Design review of the part built by this model. Coordinates are the model's own, in mm. A direction names the side the tool comes from. Round coordinates to 2 decimals unless told otherwise and drop trailing zeros. Order: outer loops, then holes, each group sorted by start corner. A loop starts at its lowest first (then second) coordinate and runs counter-clockwise, first axis right, second up.
from build123d import *

# Parameters (mm, degrees)
SKETCH1_W                 = 75
SKETCH1_H                 = 35
BOSS_EXTRUDE1_DEPTH       = 67
CUT_EXTRUDE1_DEPTH        = 60
SKETCH4_W                 = 15
SKETCH4_H                 = 10
CUT_EXTRUDE2_DEPTH        = 73.886898686
SKETCH5_W                 = 22
SKETCH5_H                 = 3
CUT_EXTRUDE3_DEPTH        = 43
F_3_0MM_DOWEL_HOLE1_D     = 3.3
F_3_0MM_DOWEL_HOLE1_DEPTH = 10
F_3_0MM_DOWEL_HOLE1_TIP   = 0.991420021
SKETCH8_R                 = 2.65
CUT_EXTRUDE4_DEPTH        = 103.079625783
FILLET1_R                 = 4


with BuildPart() as part:
    # Sketch1 → Boss-Extrude1 (new body)
    with BuildSketch(Plane.XY):
        Rectangle(SKETCH1_W, SKETCH1_H)
    extrude(amount=-BOSS_EXTRUDE1_DEPTH)

    # Sketch2 → Cut-Extrude1 (cut)
    with BuildSketch(Plane(origin=(0, 0, -67), x_dir=(-1, 0, 0), z_dir=(0, 0, -1))):
        Polygon((-22.75, -17.5), (22.75, -17.5), (22.75, 8.5), (11, 14.5), (-11, 14.5), (-22.75, 8.5), align=None)
    extrude(amount=-CUT_EXTRUDE1_DEPTH, mode=Mode.SUBTRACT)

    # Sketch4 → Cut-Extrude2 (cut, through all)
    with BuildSketch(Plane(origin=(0, 0, -7), x_dir=(-1, 0, 0), z_dir=(0, 0, -1))):
        with Locations((0, -12.5)):
            Rectangle(SKETCH4_W, SKETCH4_H)
    extrude(amount=-CUT_EXTRUDE2_DEPTH, mode=Mode.SUBTRACT)

    # Sketch5 → Cut-Extrude3 (cut)
    with BuildSketch(Plane(origin=(0, 0, -67), x_dir=(-1, 0, 0), z_dir=(0, 0, -1))):
        with Locations((0, 16)):
            Rectangle(SKETCH5_W, SKETCH5_H)
    extrude(amount=-CUT_EXTRUDE3_DEPTH, mode=Mode.SUBTRACT)

    # Ø3.0mm Dowel Hole1
    with Locations(Plane(origin=(0, 17.5, 0), x_dir=(1, 0, 0), z_dir=(0, 1, 0))):
        with Locations((-31.04375, 31), (-31.04375, 42), (-20.13125, 42), (-20.13125, 31), (-5.5, 16.36875), (5.5, 16.36875), (-5.5, 5.45625), (5.5, 5.45625), (31.04375, 42), (20.13125, 42), (31.04375, 31), (20.13125, 31)):
            Hole(F_3_0MM_DOWEL_HOLE1_D / 2, depth=F_3_0MM_DOWEL_HOLE1_DEPTH)
            with Locations((0, 0, -(F_3_0MM_DOWEL_HOLE1_DEPTH + F_3_0MM_DOWEL_HOLE1_TIP / 2))):  # 118° drill point
                Cone(0, F_3_0MM_DOWEL_HOLE1_D / 2, F_3_0MM_DOWEL_HOLE1_TIP, mode=Mode.SUBTRACT)

    # Sketch8 → Cut-Extrude4 (cut, through all)
    with BuildSketch(Plane.ZY.offset(37.5)):
        with Locations((-61, -7.5)):
            Circle(SKETCH8_R)
        with Locations((-50, -7.5)):
            Circle(SKETCH8_R)
    extrude(amount=-CUT_EXTRUDE4_DEPTH, mode=Mode.SUBTRACT)

    # Fillet1
    # the kernel refuses this fillet: 4 mm, written as the material it takes off along each edge
    with BuildSketch(Plane(origin=(33.5, 13.5, -4), x_dir=(0, 0, 1), z_dir=(1, 0, 0))) as fillet1_piece_1_section:
        Polygon((0, 0), (FILLET1_R, 0), (FILLET1_R, -FILLET1_R), (0, -FILLET1_R), align=None)
    fillet1_piece_1 = extrude(amount=FILLET1_R, mode=Mode.PRIVATE)
    fillet1_piece_1 = fillet1_piece_1 - Plane(origin=(33.5, 13.5, -4), x_dir=(0, -0.7071067811865475, -0.7071067811865475), z_dir=(1, 0, 0)) * Sphere(FILLET1_R, mode=Mode.PRIVATE)
    add(fillet1_piece_1, mode=Mode.SUBTRACT)
    with BuildSketch(Plane(origin=(-33.5, 13.5, -4), x_dir=(-1, 0, 0), z_dir=(0, 0, 1))) as fillet1_piece_2_section:
        Polygon((0, 0), (FILLET1_R, 0), (FILLET1_R, -FILLET1_R), (0, -FILLET1_R), align=None)
    fillet1_piece_2 = extrude(amount=FILLET1_R, mode=Mode.PRIVATE)
    fillet1_piece_2 = fillet1_piece_2 - Plane(origin=(-33.5, 13.5, -4), x_dir=(0.7071067811865475, -0.7071067811865475, 0), z_dir=(0, 0, 1)) * Sphere(FILLET1_R, mode=Mode.PRIVATE)
    add(fillet1_piece_2, mode=Mode.SUBTRACT)
    with BuildSketch(Plane(origin=(-33.5, 13.5, -63), x_dir=(-1, 0, 0), z_dir=(0, 0, -1))) as fillet1_piece_3_section:
        Polygon((0, 0), (FILLET1_R, 0), (FILLET1_R, FILLET1_R), (0, FILLET1_R), align=None)
    fillet1_piece_3 = extrude(amount=FILLET1_R, mode=Mode.PRIVATE)
    fillet1_piece_3 = fillet1_piece_3 - Plane(origin=(-33.5, 13.5, -63), x_dir=(0.7071067811865475, -0.7071067811865475, 0), z_dir=(0, 0, -1)) * Sphere(FILLET1_R, mode=Mode.PRIVATE)
    add(fillet1_piece_3, mode=Mode.SUBTRACT)
    with BuildSketch(Plane(origin=(33.5, 13.5, -63), x_dir=(0, 1, 0), z_dir=(1, 0, 0))) as fillet1_piece_4_section:
        Polygon((0, 0), (FILLET1_R, 0), (FILLET1_R, -FILLET1_R), (0, -FILLET1_R), align=None)
    fillet1_piece_4 = extrude(amount=FILLET1_R, mode=Mode.PRIVATE)
    fillet1_piece_4 = fillet1_piece_4 - Plane(origin=(33.5, 13.5, -63), x_dir=(0, -0.7071067811865475, 0.7071067811865475), z_dir=(1, 0, 0)) * Sphere(FILLET1_R, mode=Mode.PRIVATE)
    add(fillet1_piece_4, mode=Mode.SUBTRACT)
    with BuildSketch(Plane(origin=(37.5, -27.5, 0), x_dir=(-1, 0, 0), z_dir=(0, 1, 0)), Plane(origin=(-37.5, 13.5, 0), x_dir=(1, 0, 0), z_dir=(0, -1, 0)), Plane(origin=(37.5, -27.5, -67), x_dir=(0, 0, 1), z_dir=(0, 1, 0))) as fillet1_piece_5:
        with BuildLine():
            CenterArc((FILLET1_R, -FILLET1_R), FILLET1_R, 90, 90)
            Line((0, -FILLET1_R), (0, 0))
            Line((0, 0), (FILLET1_R, 0))
        make_face()
    extrude(amount=41, mode=Mode.SUBTRACT)
    with BuildSketch(Plane(origin=(-37.5, 13.5, -67), x_dir=(1, 0, 0), z_dir=(0, -1, 0))) as fillet1_piece_6:
        with BuildLine():
            CenterArc((FILLET1_R, FILLET1_R), FILLET1_R, 180, 90)
            Line((0, FILLET1_R), (0, 0))
            Line((0, 0), (FILLET1_R, 0))
        make_face()
    extrude(amount=41, mode=Mode.SUBTRACT)
    with BuildSketch(Plane(origin=(-1, 17.5, -67), x_dir=(0, -1, 0), z_dir=(-1, 0, 0))) as fillet1_piece_7:
        with BuildLine():
            CenterArc((FILLET1_R, FILLET1_R), FILLET1_R, 180, 90)
            Line((0, FILLET1_R), (0, 0))
            Line((0, 0), (FILLET1_R, 0))
        make_face()
    extrude(amount=32.5, mode=Mode.SUBTRACT)
    with BuildSketch(Plane(origin=(33.5, 17.5, -67), x_dir=(0, 0, 1), z_dir=(-1, 0, 0))) as fillet1_piece_8:
        with BuildLine():
            CenterArc((FILLET1_R, -FILLET1_R), FILLET1_R, 90, 90)
            Line((0, -FILLET1_R), (0, 0))
            Line((0, 0), (FILLET1_R, 0))
        make_face()
    extrude(amount=32.5, mode=Mode.SUBTRACT)
    with BuildSketch(Plane(origin=(37.5, 17.5, -4), x_dir=(-1, 0, 0), z_dir=(0, 0, -1)), Plane(origin=(-37.5, 17.5, -4), x_dir=(0, -1, 0), z_dir=(0, 0, -1))) as fillet1_piece_9:
        with BuildLine():
            CenterArc((FILLET1_R, -FILLET1_R), FILLET1_R, 90, 90)
            Line((0, -FILLET1_R), (0, 0))
            Line((0, 0), (FILLET1_R, 0))
        make_face()
    extrude(amount=59, mode=Mode.SUBTRACT)
    with BuildSketch(Plane(origin=(33.5, 17.5, 0), x_dir=(0, -1, 0), z_dir=(-1, 0, 0))) as fillet1_piece_10:
        with BuildLine():
            CenterArc((FILLET1_R, -FILLET1_R), FILLET1_R, 90, 90)
            Line((0, -FILLET1_R), (0, 0))
            Line((0, 0), (FILLET1_R, 0))
        make_face()
    extrude(amount=67, mode=Mode.SUBTRACT)


solid = part.part
1) Take a section at D-D on y = 3.5. Give the boundary of the cut face in (x, z).
Results:
outline: (-37.5, -63) arc R4 ccw to (-33.5, -67) - (-22.75, -67) - (-22.75, -7) - (22.75, -7) - (22.75, -67) - (33.5, -67) arc R4 ccw to (37.5, -63) - (37.5, -4) arc R4 ccw to (33.5, 0) - (-33.5, 0) arc R4 ccw to (-37.5, -4) - close
2) To check wall thickness, follow line 1 along X through (y, z) = (-7, -39.5); line 2 along X through (y, z) = (8, -43.5); line 3 along Z through (x, y) = (-31, -6). State the ranges of each line that lie inside material, in increasing order.
Results:
line 1: x = -37.5 to -22.75, 22.75 to 37.5
line 2: x = -37.5 to -31.73, -30.36 to -22.75, 22.75 to 30.36, 31.73 to 37.5
line 3: z = -67 to -63.18, -58.82 to -52.18, -47.82 to 0
3) For faces 1 (the face through (16.793, 11.542, -37.42)), 2 (the face through (11, 16, -46)), 3 (the face through (7.5, -13, -4)), list the 3-axis set-ups (+Z, -Z, +X, -X, +Y, -Y) from which the entire face can be reached by the end or side of a thin tool; tool diameter is ignored.
Results:
face 1: -Z, -Y
face 2: -Z, +Y, -Y
face 3: +Z, -Z, -Y
4) Take a section at B-B on z = -61. Give the boundary of the cut face in (x, y), plus the area to 3 significant figures.
Results:
outline: (-37.5, -17.5) - (-22.75, -17.5) - (-22.75, -10.15) - (-37.5, -10.15) - close; (-37.5, -4.85) - (-22.75, -4.85) - (-22.75, 8.5) - (-11, 14.5) - (-11, 17.5) - (-33.5, 17.5) arc R4 ccw to (-37.5, 13.5) - close; (11, 14.5) - (22.75, 8.5) - (22.75, -4.85) - (37.5, -4.85) - (37.5, 13.5) arc R4 ccw to (33.5, 17.5) - (11, 17.5) - close; (22.75, -17.5) - (37.5, -17.5) - (37.5, -10.15) - (22.75, -10.15) - close
area: 1,010 mm2
5) The part is to be moulded in two halves that separate along Y. For faces 4 (the face through (5.63, 6.68, -5.2)), 5 (the face through (-30.23, -8.51, -58.55)), 6 (the face through (0, -1, -7)), say which applies: released by +Y, released by -Y, zero draft, split by the parting line, or undercut.
Results:
face 4: released by +Y
face 5: undercut
face 6: zero draft
6) Clearance check with flat-ended pins moving along their axes: P1, Ø3.5, axis at y = 16, z = -45.5, coming from the -X side; P2, Ø2.5, axis at x = -20.13, z = -42, coming from the -Y side; P3, Ø3.5, axis at x = 0.5, y = 16, coming from the -Z side; P4, Ø2, axis at x = 5.5, z = -5.46, coming from the +Y side. State where each tip first meets the part, or that it passes through.
Results:
P1: stops at x = -37.43
P2: passes through
P3: stops at z = -24
P4: stops at y = 7.11
7) Take a section at A-A on y = -14. Give the boundary of the cut face in (x, z), plus the area to 3 significant figures.
Results:
outline: (-37.5, -63) arc R4 ccw to (-33.5, -67) - (-22.75, -67) - (-22.75, -7) - (-7.5, -7) - (-7.5, 0) - (-33.5, 0) arc R4 ccw to (-37.5, -4) - close; (7.5, -7) - (22.75, -7) - (22.75, -67) - (33.5, -67) arc R4 ccw to (37.5, -63) - (37.5, -4) arc R4 ccw to (33.5, 0) - (7.5, 0) - close
area: 2,180 mm2
8) Take a section at C-C on x = 25. Give the boundary of the cut face in (y, z).
Results:
outline: (-17.5, -67) - (13.5, -67) arc R4 ccw to (17.5, -63) - (17.5, -4) arc R4 ccw to (13.5, 0) - (-17.5, 0) - close; hole circle Ø5.3 at (-7.5, -61); hole circle Ø5.3 at (-7.5, -50)
